from build123d import *

# Parameters (mm, degrees)
BASE_DEPTH           = 20
SKETCH2_R            = 1.4
SCREW_HOLES_DEPTH    = 30.681644159
SKETCH3_W            = 10
SKETCH3_H            = 8
SKETCH3_W_2          = 5
SKETCH3_H_2          = 3
ZIP_TIE_SLOTS_DEPTH  = 9
F_1MM_EDGE_FILLETS_R = 1


with BuildPart() as part:
    # Sketch1 → Base (new body)
    with BuildSketch(Plane(origin=(0, 0, 0), x_dir=(1, 0, 0), z_dir=(0, 1, 0))):
        with BuildLine():
            Line((9, 20), (9, 15.5))
            ThreePointArc((9, 15.5), (7.797918472, 15.002081528), (7.3, 13.8))
            Line((7.3, 13.8), (7.3, 11.2))
            ThreePointArc((7.3, 11.2), (7.797918472, 9.997918472), (9, 9.5))
            Line((9, 9.5), (9, -9.5))
            ThreePointArc((9, -9.5), (7.797918472, -9.997918472), (7.3, -11.2))
            Line((7.3, -11.2), (7.3, -13.8))
            ThreePointArc((7.3, -13.8), (7.797918472, -15.002081528), (9, -15.5))
            Line((9, -15.5), (9, -20))
            Line((9, -20), (0, -20))
            Line((0, -20), (0, 20))
            Line((0, 20), (9, 20))
        make_face()
    extrude(amount=BASE_DEPTH)

    # Sketch2 → Screw Holes (cut, through all)
    with BuildSketch(Plane(origin=(9, 0, 0), x_dir=(0, 0, -1), z_dir=(1, 0, 0))):
        with Locations((-5, 15)):
            Circle(SKETCH2_R)
        with Locations((5, 15)):
            Circle(SKETCH2_R)
        with Locations((5, 5)):
            Circle(SKETCH2_R)
        with Locations((-5, 5)):
            Circle(SKETCH2_R)
    extrude(amount=-SCREW_HOLES_DEPTH, mode=Mode.SUBTRACT)

    # Sketch3 → Zip Tie Slots (add)
    # profile 1 of 2: a face of its own
    with BuildSketch(Plane(origin=(0, 0, 0), x_dir=(0, 0, -1), z_dir=(1, 0, 0))):
        with Locations((-25, 10)):
            Rectangle(SKETCH3_W, SKETCH3_H)
        with Locations((-25, 10)):
            Rectangle(SKETCH3_W_2, SKETCH3_H_2, mode=Mode.SUBTRACT)
    # profile 2 of 2: a face of its own
    with BuildSketch(Plane(origin=(0, 0, 0), x_dir=(0, 0, -1), z_dir=(1, 0, 0))):
        with Locations((25, 10)):
            Rectangle(SKETCH3_W, SKETCH3_H)
        with Locations((25, 10)):
            Rectangle(SKETCH3_W_2, SKETCH3_H_2, mode=Mode.SUBTRACT)
    extrude(amount=ZIP_TIE_SLOTS_DEPTH)

    # 1mm Edge Fillets
    f_1mm_edge_fillets_edges = [part.edges().sort_by_distance(p)[0] for p in [
        (4.5, 0, -20),
        (4.5, 0, 20),
        (0, 0, 0),
        (0, 17, -20),
        (0, 17, 20),
        (4.5, 20, -20),
        (0, 20, 0),
        (0, 3, 20),
        (4.5, 6, 20),
        (4.5, 14, 20),
        (0, 14, 25),
        (4.5, 14, 30),
        (4.5, 6, 30),
        (0, 6, 25),
        (0, 3, -20),
        (4.5, 14, -20),
        (4.5, 6, -20),
        (0, 6, -25),
        (4.5, 6, -30),
        (0, 10, -30),
        (4.5, 14, -30),
        (0, 14, -25),
        (4.5, 20, 20),
    ]]
    fillet(f_1mm_edge_fillets_edges, radius=F_1MM_EDGE_FILLETS_R)


solid = part.part
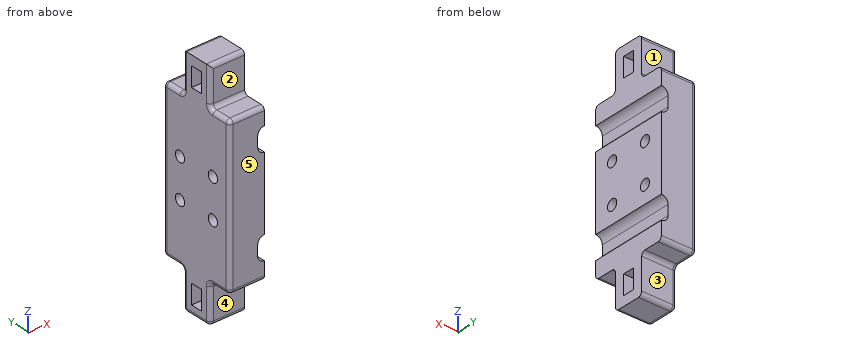
Read the model definition and answer for the solid it produces. Units are mm, in the model's axes. Face numbers are marked on the shaded views. A direction names the side the tool comes from. Coordinates: 2 decimals unless noted, no trailing zeros. Order: outer loops, then holes, each group sorted by start corner. A loop starts at its lowest first (then second) coordinate and runs counter-clockwise, first axis right, second up. Notation, with made-up numbers: M 31.25,16.5 L 72.25,16.5 A23 cw 72.25,49.5 Z; hole C 31.25,31.5 d2. An arc over 180 degrees is marked long. Put each result on its own line as item: value. Start each with the question number.
Item 1: Section D-D, the plane x = 8 is taken. Count the separate pieces of the cut face and the enclosed holes in it, plus the area to 3 significant figures.
Item 2: Consider probe 1 along Y at (x, z) = (5.5, -5); probe 2 along Y at (x, z) = (5.75, 25); probe 3 along Y at (x, z) = (2, 5.5). Determine where each line is inside the solid, lowest interval first. Write a range as [from, to].
Item 3: Given pin 1 Ø3 at (x, y) = (6, 3.5) entering from -Z; pin 2 Ø2 at (x, z) = (2, -20.5) entering from -Y; pin 3 Ø4 at (x, z) = (3.5, -24.5) entering from +Y, each flat-ended and moving along its own axis, determine where each tip first touches the part or whether it passes through.
Item 4: For the marked faces 1, 2, 3, 4 and 5, determine the directions among +Z, -Z, +X, -X, +Y, -Y from which every point of the face is accessible in a straight line to the end or side of a thin tool.
Item 5: Section C-C, the plane z = 5 is taken. Determine the outline of the cut face in (x, y), plus the area to 3 significant figures.
Item 6: Section B-B, the plane z = -26 is taken. Determine the outline of the cut face in (x, y), plus the area to 3 significant figures.
Item 7: Section A-A, the plane y = 10 is taken. Determine the outline of the cut face in (x, z).
Computed:
1. separate pieces: 3
1. enclosed holes: 6
1. area: 691 mm2
2. probe 1: y = [0, 3.6], [6.4, 13.6], [16.4, 20]
2. probe 2: y = [6, 8.5], [11.5, 14]
2. probe 3: y = [0, 3.69], [6.31, 13.69], [16.31, 20]
3. pin 1: stops at z = -20
3. pin 2: stops at y = 0.13
3. pin 3: stops at y = 14
4. face 1: +Z, +X, -X, +Y
4. face 2: +Z, +X, -X, -Y
4. face 3: -Z, +X, -X, +Y
4. face 4: -Z, +X, -X, -Y
4. face 5: +Z, -Z, +X, -X, -Y
5. outline: M 0,1 A1 ccw 1,0 L 9,0 L 9,3.6 L 0,3.6 Z; M 0,6.4 L 9,6.4 L 9,13.6 L 0,13.6 Z; M 0,16.4 L 9,16.4 L 9,20 L 1,20 A1 ccw 0,19 Z
5. area: 129 mm2
6. outline: M 0,7 A1 ccw 1,6 L 9,6 L 9,8.5 L 0,8.5 Z; M 0,11.5 L 9,11.5 L 9,14 L 1,14 A1 ccw 0,13 Z
6. area: 44.6 mm2
7. outline: M 0,-29 A1 ccw 1,-30 L 9,-30 L 9,-27.5 L 0,-27.5 Z; M 0,-22.5 L 9,-22.5 L 9,-15.5 A1.7 cw 7.3,-13.8 L 7.3,-11.2 A1.7 cw 9,-9.5 L 9,9.5 A1.7 cw 7.3,11.2 L 7.3,13.8 A1.7 cw 9,15.5 L 9,22.5 L 0,22.5 Z; M 0,27.5 L 9,27.5 L 9,30 L 0,30 Z
